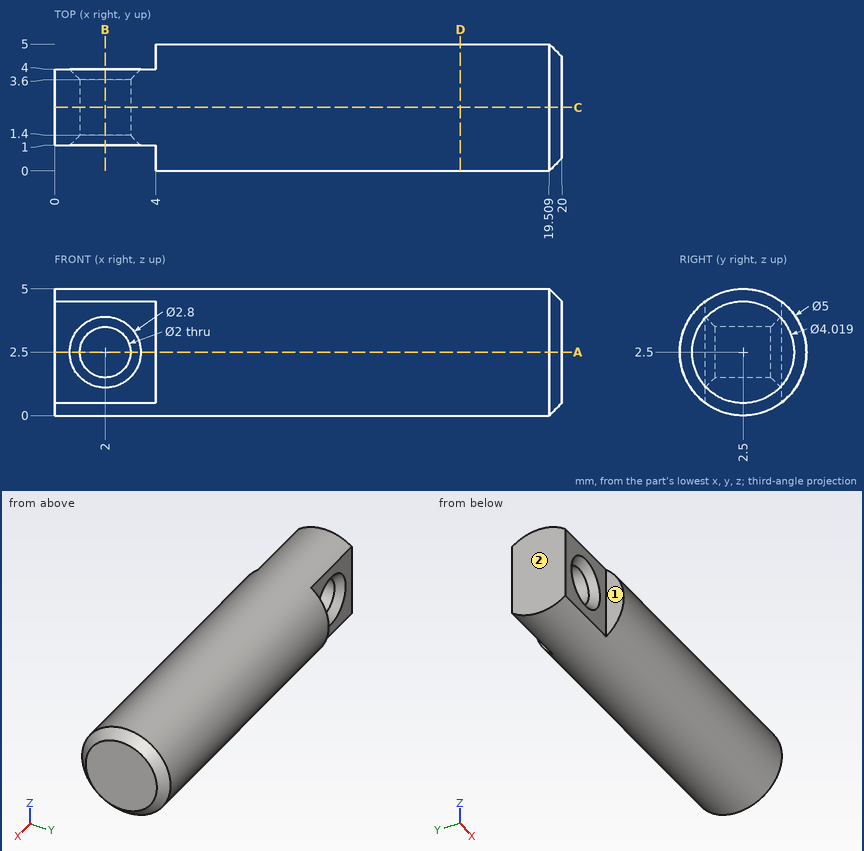
Part print with two shaded views. Sizes in mm from the minimum x, y, z corner. A direction names the side the tool comes from. Coordinates: 2 decimals unless noted, no trailing zeros. Loops run counter-clockwise (first coordinate to the right, second up) from the corner with the lowest first, then second, coordinate; pieces in that order, holes last. Notation, with made-up numbers: (72, 13) -> (87, 13) arc R18 ccw to (87, 36) -> close; hole circle Ø9 at (80.25, -18). An arc over 180 degrees is marked (long way). Answer as a JSON object with one key per item and string values.
Q1. Probe probe 1 along X at (y, z) = (2.6, 2.5); probe 2 along Z at (x, y) = (2, 1.9); probe 3 along Y at (x, z) = (8.75, 1). List the from-to ranges inside material, lowest first.
Report:
{"probe 1": "x = 0 to 1, 3 to 20", "probe 2": "z = 0.07 to 1.5, 3.5 to 4.93", "probe 3": "y = 0.5 to 4.5"}
Q2. Flat gauge pins, fed straight in: P1, Ø3, axis at x = 1, z = 2, coming from the -Y side; P2, Ø1.2, axis at x = 2, z = 2.5, coming from the +Y side; P3, Ø1.5, axis at x = 5.5, y = 1.5, coming from the -Z side; P4, Ø2, axis at x = 11, z = 1, coming from the +Y side. Where does each tip first touch, or does it go through?
Report:
{"P1": "stops at y = 1", "P2": "passes through", "P3": "stops at z = 0.01", "P4": "stops at y = 4.95"}
Q3. Cut at D-D (x = 16). List the corners of the cut face in (y, z).
Report:
{"outline": "circle Ø5 at (2.5, 2.5)"}
Q4. Cut at A-A (z = 2.5). List the corners of the cut face in (x, y).
Report:
{"outline": "(0, 1) -> (0.6, 1) -> (1, 1.4) -> (1, 3.6) -> (0.6, 4) -> (0, 4) -> close; (3, 1.4) -> (3.4, 1) -> (4, 1) -> (4, 0) -> (19.51, 0) -> (20, 0.49) -> (20, 4.51) -> (19.51, 5) -> (4, 5) -> (4, 4) -> (3.4, 4) -> (3, 3.6) -> close"}
Q5. Cut at B-B (x = 2). List the corners of the cut face in (y, z).
Report:
{"outline": "(1, 0.5) arc R2.5 ccw to (4, 0.5) -> (4, 1.1) -> (3.6, 1.5) -> (1.4, 1.5) -> (1, 1.1) -> close; (1, 3.9) -> (1.4, 3.5) -> (3.6, 3.5) -> (4, 3.9) -> (4, 4.5) arc R2.5 ccw to (1, 4.5) -> close"}
Q6. 3-axis set-ups, long thin cutter, end or side, ignore diameter. For the marked faces 1 and 2: which of +Z, -Z, +X, -X, +Y, -Y reach the whole face in a straight line?
Report:
{"face 1": "+Z, -Z, -X, -Y", "face 2": "+Z, -Z, -X, +Y, -Y"}
Q7. Cut at C-C (y = 2.5). List the corners of the cut face in (x, z).
Report:
{"outline": "(0, 0) -> (19.51, 0) -> (20, 0.49) -> (20, 4.51) -> (19.51, 5) -> (0, 5) -> close; hole circle Ø2 at (2, 2.5)"}
